For this review, take the finished solid that the model builds, in its own axes (mm). A direction names the side the tool comes from. Give positions to 0.01 mm unless a question says otherwise; leave off trailing zeros. Write each loop counter-clockwise with the first axis right and the second up, starting at its lowest first coordinate (ties: lowest second). Pieces come first, ordered by that corner, then holes. Notation, with made-up numbers: (-28.75, 18) -> (-1.75, 18) arc R26 cw to (-1.75, 48) -> close; hole circle Ø5 at (22.5, -30). An arc over 180 degrees is marked (long way). Return JSON: item names as keys, results as strings.
from build123d import *

# Parameters (mm, degrees)
SCHIZZO2_R                   = 9
ESTRUSIONE_ESTRUSIONE1_DEPTH = 135
SCHIZZO3_R                   = 16
ESTRUSIONE_ESTRUSIONE2_DEPTH = 20
TAGLIO_ESTRUSIONE1_REACH     = 161.075
SCHIZZO4_R                   = 3
SMUSSO1_SIZE                 = 3
SMUSSO2_SIZE                 = 2
TAGLIO_ESTRUSIONE2_START     = -1.3
SCHIZZO6_R                   = 9
SCHIZZO6_R_2                 = 8.15
TAGLIO_ESTRUSIONE2_DEPTH     = 1.3


with BuildPart() as part:
    # Schizzo2 → Estrusione-Estrusione1 (new body)
    with BuildSketch(Plane.XY):
        Circle(SCHIZZO2_R)
    extrude(amount=ESTRUSIONE_ESTRUSIONE1_DEPTH)

    # Schizzo3 → Estrusione-Estrusione2 (add)
    with BuildSketch(Plane.XY.offset(135)):
        Circle(SCHIZZO3_R)
    extrude(amount=ESTRUSIONE_ESTRUSIONE2_DEPTH)

    # Schizzo4 → Taglio-Estrusione1 (cut, up to next)
    with BuildSketch(Plane(origin=(0, 16, 0), x_dir=(1, 0, 0), z_dir=(0, 1, 0)), mode=Mode.PRIVATE) as taglio_estrusione1_sk1:
        with Locations(Location((0, -145, 0), (0, 0, 270))):
            Circle(SCHIZZO4_R)
    taglio_estrusione1_tool1 = extrude(taglio_estrusione1_sk1.sketch, amount=-TAGLIO_ESTRUSIONE1_REACH, mode=Mode.PRIVATE) & part.part
    add(taglio_estrusione1_tool1.solids().sort_by_distance((0, 16, 145))[0], mode=Mode.SUBTRACT)

    # Smusso1
    smusso1_edges = [part.edges().sort_by_distance(p)[0] for p in [
        (-16, 0, 135),
        (-16, 0, 155),
    ]]
    chamfer(smusso1_edges, length=SMUSSO1_SIZE)

    # Smusso2
    smusso2_edges = [part.edges().sort_by_distance(p)[0] for p in [
        (-9, 0, 0),
    ]]
    chamfer(smusso2_edges, length=SMUSSO2_SIZE)

    # Schizzo6 → Taglio-Estrusione2 (cut)
    with BuildSketch(Plane.XY.offset(83.5).offset(TAGLIO_ESTRUSIONE2_START)):
        Circle(SCHIZZO6_R)
        Circle(SCHIZZO6_R_2, mode=Mode.SUBTRACT)
    taglio_estrusione2 = extrude(amount=TAGLIO_ESTRUSIONE2_DEPTH, mode=Mode.SUBTRACT)

    # Specchia1: Taglio-Estrusione2 across plane
    add(taglio_estrusione2.mirror(Plane(origin=(0, 0, 72.3), x_dir=(1, 0, 0), z_dir=(0, 0, -1))), mode=Mode.SUBTRACT)


solid = part.part
1. For faces 1 (the cylindrical face through (-1.172, 8.923, 72.161)), 2 (the flat face through (0, 0, 155)), 3 (the cylindrical face through (-6.468, -4.959, 61.759)), list the 3-axis set-ups (+Z, -Z, +X, -X, +Y, -Y) from which the entire face can be reached by the end or side of a thin tool; tool diameter is ignored.
Results found:
{"face 1": "-Z", "face 2": "+Z, +X, -X, +Y, -Y", "face 3": "none"}
2. Add section D-D, the plane z = 145. State the section outline as (x, y) points.
Results found:
{"outline": "(-3, -15.72) -> (-3, 15.72) arc R16 ccw to start; (3, -15.72) arc R16 ccw to (3, 15.72) -> close"}
3. To check wall thickness, follow probe 1 along Z at (x, y) = (0, -3.5); probe 2 along Z at (x, y) = (10, -6); probe 3 along X at (y, z) = (2, 145). State the ranges of each line that lie inside material, in increasing order.
Results found:
{"probe 1": "z = 0 to 142, 148 to 155", "probe 2": "z = 135 to 155", "probe 3": "x = -15.87 to -3, 3 to 15.87"}
4. Add section C-C, the plane z = 76. State the section outline as (x, y) points, plus the area to 3 significant figures.
Results found:
{"outline": "circle Ø18 at (0, 0)", "area": "254 mm²"}
5. For pin 1 (3.5 mm diameter, centred on x = 0, z = 145, fed in from +Y); pin 2 (6 mm diameter, centred on x = 2, z = 32.5, fed in from -Y); pin 3 (8 mm diameter, centred on y = 9.5, z = 40, fed in from -X); pin 4 (10 mm diameter, centred on x = 10.5, z = 121.5, fed in from -Y), all flat-tipped, find the tip position at first contact; note any pin that passes through.
Results found:
{"pin 1": "passes through", "pin 2": "stops at y = -9", "pin 3": "stops at x = -7.12", "pin 4": "stops at y = -7.12"}
6. The part is to be moulded in two halves that separate along Z. For faces 4 (the flat face through (-5, 7, 62.4)), 5 (the cylindrical face through (-1.172, 8.923, 108.89)), 6 (the flat face through (0, 0, 0)), say which applies: +Z half, -Z half, draft (parallel to the pull), parting line (faces both ways), or undercut.
Results found:
{"face 4": "undercut", "face 5": "draft", "face 6": "-Z half"}
